Geometry check sheet. Reference: the model listing, model coordinates, mm. A direction names the side the tool comes from. Coordinates: 2 decimals unless noted, no trailing zeros. Loops run counter-clockwise (first coordinate to the right, second up) from the corner with the lowest first, then second, coordinate; pieces in that order, holes last. Notation, with made-up numbers: (-15.5, -36.5) - (23.5, -36.5) arc R9 cw to (23.5, -20.5) - close; hole circle Ø10 at (-36, 44). An arc over 180 degrees is marked (long way). Write item = value, one per line. Start each with the question number.
Autodesk Inventor part; units mm, degrees
ref_plane "Work Plane1" through (0, 0, 0) normal (0, -1, 0) x (1, 0, 0)
ref_plane "YZ Plane" through (0, 0, 0) normal (1, 0, 0) x (0, 1, 0)
ref_plane "XZ Plane" through (0, 0, 0) normal (0, 1, 0) x (-1, 0, 0)
sketch "Sketch1" plane through (0, 0, 0) normal (0, 0, 1) x (1, 0, 0)
  line L0 (-9, 0) -> (54, 0) construction
  line L1 (0, -13.86) -> (0, 13.86) construction
  line L2 (0, 8.5) -> (41, 8.5)
  line L3 (41, 8.5) -> (41, -8.5)
  line L4 (41, -8.5) -> (0, -8.5)
  line L5 (0, -9.9) -> (45, -9.9)
  line L6 (45, -9.9) -> (45, 9.9)
  line L7 (45, 9.9) -> (0, 9.9)
  line L8 (0, 8.5) -> (0, 9.9)
  line L9 (0, -8.5) -> (0, -9.9)
  point P0 (0, 0)
  dimension "d0" = 17
  dimension "d1" = 19.8
  dimension "d2" = 45
  dimension "d3" = 4
extrude "Extrusion1" add sketch "Sketch1" along normal blind 9.5
sketch "Sketch2" plane through (45, -9.9, 0) normal (1, 0, 0) x (0, 0, -1)
  line L0 (0, 0) -> (0, 19.8) construction
  line L1 (0, 19.8) -> (-9.5, 19.8) construction
  line L2 (-9.5, 0) -> (-9.5, 19.8) construction
  line L3 (0, 0) -> (-9.5, 0) construction
  line L4 (-9.5, 0) -> (-9.5, 19.8) construction
  line L5 (-9.5, 9.9) -> (0, 9.9) construction
  line L6 (0, 0) -> (-9.5, 0) construction
  line L7 (-4.75, 0) -> (-4.75, 19.8) construction
  circle A0 centre (-4.75, 9.9) radius 2.5
  dimension "d6" = 5
extrude "Extrusion2" add sketch "Sketch2" along normal blind 9.5
ref_plane "Work Plane1" through (0, 0, 0) normal (0, -1, 0) x (1, 0, 0)
sketch "Sketch3" plane through (0, 0, 0) normal (0, -1, 0) x (1, 0, 0)
  line L0 (54.5, 2.25) -> (54.5, 7.25) construction
  line L1 (-11.7, 4.75) -> (70.2, 4.75) construction
  line L2 (54.5, 2.25) -> (54.5, 7.25) construction
  line L3 (45, 7.25) -> (45, 2.25) construction
  arc A0 (50, 4.75) -> (59, 4.75) centre (54.5, 4.75) ccw
  line L4 (59, 4.75) -> (50, 4.75)
  point P0 (0, 0)
  dimension "d9" = 4.5
revolve "Revolution1" add sketch "Sketch3" angle 360 about axis through (45, 0, 4.75) along (1, 0, 0)
fillet "Fillet1" radius 1 1 edges at (45, 0, 7.25)
fillet "Fillet2" radius 2 2 edges at (41, -8.5, 4.75) (41, 8.5, 4.75)
fillet "Fillet3" radius 0.5 22 edges at (22.5, 9.9, 9.5) (41, 0, 9.5) (19.5, -8.5, 9.5) (19.5, 8.5, 9.5) (41, 0, 0) (19.5, -8.5, 0) (19.5, 8.5, 0) (0, 9.2, 0) (0, 9.2, 9.5) (0, -9.2, 9.5) (0, -9.2, 0) (0, -9.9, 4.75) (0, -8.5, 4.75) (22.5, -9.9, 9.5) (22.5, -9.9, 0) (0, 9.9, 4.75) (0, 8.5, 4.75) (45, 9.9, 4.75) (45, 0, 9.5) (45, -9.9, 4.75) (45, 0, 0) (22.5, 9.9, 0)
properties part number "10x20-plunger-V1"
(1) Sectioned sample at A-A on x = 10. Enter the section's corners in (y, z).
(2) Scan lines: line 1 (Y direction, x = 19, z = 5); line 2 (X direction, y = 5.25, z = 6); line 3 (X direction, y = -2.25, z = 7). Record each from-to range of solid material in increasing order.
(3) Sectioned sample at B-B on z = 4.75. Enter the section's corners in (x, y).
(4) Tool access check on faces 4 (the face through (23, 9.9, 5)), 5 (the face through (41, 0, 5)). Record the directions out of +Z, -Z, +X, -X, +Y, -Y that give a thin tool (end or side, any length) a straight path to the whole face; none if there is none.
(5) Sectioned sample at D-D on x = 47. Enter the section's corners in (y, z).
(6) Depth check by flat-ended pin: pin 1 (1 mm diameter, centred on y = -7.5, z = 4.5, fed in from +X); pin 2 (6 mm diameter, centred on x = 27, y = 5, fed in from +Z); pin 3 (2.5 mm diameter, centred on y = -1.5, z = 4.5, fed in from -X); pin 4 (2 mm diameter, centred on x = 49, z = 2.5, fed in from +Y). Enter the tip coordinate at first touch or a pass-through.
(7) Draft check along Y on faces 1 (the face through (40.43, 7.9, 4.81)), 2 (the face through (22, -9.9, 5)), 3 (the face through (48.346, -0.751, 2.365)). Enter one of: pulls with the +Y half, pulls with the -Y half, needs draft (parallel to the pull), parting line crosses it, or undercut.
(8) Sectioned sample at C-C on y = 0. Enter the section's corners in (x, z), plus the area to 3 significant figures.
Working result:
q1.outline = (-9.9, 0.5) arc R0.5 ccw to (-9.4, 0) - (-9, 0) arc R0.5 ccw to (-8.5, 0.5) - (-8.5, 9) arc R0.5 ccw to (-9, 9.5) - (-9.4, 9.5) arc R0.5 ccw to (-9.9, 9) - close; (8.5, 0.5) arc R0.5 ccw to (9, 0) - (9.4, 0) arc R0.5 ccw to (9.9, 0.5) - (9.9, 9) arc R0.5 ccw to (9.4, 9.5) - (9, 9.5) arc R0.5 ccw to (8.5, 9) - close
q2.line_1 = -9.9 to -8.5, 8.5 to 9.9
q2.line_2 = 41 to 45
q2.line_3 = 41 to 45.05, 51.32 to 57.68
q3.outline = (0, -9.4) arc R0.5 ccw to (0.5, -9.9) - (44.5, -9.9) arc R0.5 ccw to (45, -9.4) - (45, -3.5) arc R1 cw to (46, -2.5) - (50.76, -2.5) arc R4.5 ccw (long way) to (50.76, 2.5) - (46, 2.5) arc R1 cw to (45, 3.5) - (45, 9.4) arc R0.5 ccw to (44.5, 9.9) - (0.5, 9.9) arc R0.5 ccw to (0, 9.4) - (0, 9) arc R0.5 ccw to (0.5, 8.5) - (39, 8.5) arc R2 cw to (41, 6.5) - (41, -6.5) arc R2 cw to (39, -8.5) - (0.5, -8.5) arc R0.5 ccw to (0, -9) - close
q4.face_4 = +Z, -Z, +X, -X, +Y
q4.face_5 = +Z, -Z, -X
q5.outline = circle Ø5 at (0, 4.75)
q6.pin_1 = 45
q6.pin_2 = through
q6.pin_3 = 41
q6.pin_4 = 2.17
q7.face_1 = undercut
q7.face_2 = pulls with the -Y half
q7.face_3 = parting line crosses it
q8.outline = (41, 0.5) arc R0.5 ccw to (41.5, 0) - (44.5, 0) arc R0.5 ccw to (45, 0.5) - (45, 1.25) arc R1 cw to (46, 2.25) - (50.76, 2.25) arc R4.5 ccw (long way) to (50.76, 7.25) - (46, 7.25) arc R1 cw to (45, 8.25) - (45, 9) arc R0.5 ccw to (44.5, 9.5) - (41.5, 9.5) arc R0.5 ccw to (41, 9) - close
q8.area = 128 mm2
